from build123d import *

# Parameters (mm, degrees)
SKETCH1_W           = 10
SKETCH1_H           = 3
SKETCH1_W_2         = 3
SKETCH1_H_2         = 10
SKETCH1_R           = 3.25
BOSS_EXTRUDE1_DEPTH = 3


with BuildPart() as part:
    # Sketch1 → Boss-Extrude1 (new body)
    with BuildSketch(Plane.XY):
        Polygon((-112.631023813, -53.728350242), (-112.631023813, -63.840272517), (-112.631023813, -85.840272517), (119.257053912, -85.840272517), (137.368976187, -67.728350242), (187.368976187, -17.728350242), (137.368976187, 32.271649758), (137.368976187, 22.271649758), (134.368976187, 22.271649758), (134.368976187, 32.271649758), (60.378976187, 32.271649758), (60.378976187, 26.271649758), (57.378976187, 26.271649758), (57.378976187, 32.271649758), (42.378976187, 32.271649758), (27.378976187, 32.271649758), (27.378976187, 26.271649758), (24.378976187, 26.271649758), (24.378976187, 32.271649758), (-62.631023813, 32.271649758), (-109.631023813, 32.271649758), (-109.631023813, 22.271649758), (-112.631023813, 22.271649758), (-112.631023813, 12.271649758), (-109.631023813, 12.271649758), (-109.631023813, 2.271649758), (-112.631023813, 2.271649758), (-112.631023813, -7.728350242), (-109.631023813, -7.728350242), (-109.631023813, -17.728350242), (-112.631023813, -17.728350242), (-112.631023813, -27.728350242), (-109.631023813, -27.728350242), (-109.631023813, -50.728350242), (-102.631023813, -50.728350242), (-102.631023813, -53.728350242), align=None)
        with Locations((-87.631023813, -52.228350242)):
            Rectangle(SKETCH1_W, SKETCH1_H, mode=Mode.SUBTRACT)
        with Locations((-67.631023813, -52.228350242)):
            Rectangle(SKETCH1_W, SKETCH1_H, mode=Mode.SUBTRACT)
        with Locations((-47.631023813, -52.228350242)):
            Rectangle(SKETCH1_W, SKETCH1_H, mode=Mode.SUBTRACT)
        with Locations((-27.631023813, -52.228350242)):
            Rectangle(SKETCH1_W, SKETCH1_H, mode=Mode.SUBTRACT)
        with Locations((-7.631023813, -52.228350242)):
            Rectangle(SKETCH1_W, SKETCH1_H, mode=Mode.SUBTRACT)
        with Locations((12.368976187, -52.228350242)):
            Rectangle(SKETCH1_W, SKETCH1_H, mode=Mode.SUBTRACT)
        Polygon((27.368976187, -50.728350242), (37.371405326, -50.728350242), (37.368976187, -53.728350242), (27.368976187, -53.728350242), align=None, mode=Mode.SUBTRACT)
        Polygon((107.3787447, -50.728350242), (117.381121881, -50.728350242), (117.369073889, -53.728350242), (107.369073889, -53.728350242), align=None, mode=Mode.SUBTRACT)
        Polygon((127.381202522, -50.728350242), (137.381202522, -50.728350242), (137.36915453, -53.728350242), (127.36915453, -53.728350242), align=None, mode=Mode.SUBTRACT)
        with Locations((135.868976187, -32.728350242)):
            Rectangle(SKETCH1_W_2, SKETCH1_H_2, mode=Mode.SUBTRACT)
        with Locations((-57.669534365, 17.271649758)):
            Circle(SKETCH1_R, mode=Mode.SUBTRACT)
        with Locations((135.868976187, -12.728350242)):
            Rectangle(SKETCH1_W_2, SKETCH1_H_2, mode=Mode.SUBTRACT)
        with Locations((152.368976187, -17.728350242)):
            Rectangle(SKETCH1_W, SKETCH1_H, mode=Mode.SUBTRACT)
        with Locations((172.368976187, -17.728350242)):
            Rectangle(SKETCH1_W, SKETCH1_H, mode=Mode.SUBTRACT)
        with Locations((135.868976187, 7.271649758)):
            Rectangle(SKETCH1_W_2, SKETCH1_H_2, mode=Mode.SUBTRACT)
    extrude(amount=BOSS_EXTRUDE1_DEPTH)


solid = part.part
Build history of the part. All positions in model axes, mm. Round coordinates to 2 decimals unless told otherwise and drop trailing zeros. Loops run counter-clockwise (first coordinate to the right, second up) from the corner with the lowest first, then second, coordinate; pieces in that order, holes last. Notation, with made-up numbers: (29, 84.5) -> (84, 84.5) arc R5 ccw to (84, 90.5) -> close; hole circle Ø8 at (-8.5, -34). An arc over 180 degrees is marked (long way). One line per item, written item: value. Start each with the question number.
Q1. Drop flat-ended pins along their axis: pin 1 Ø1.5 at (x, z) = (130.5, 2) entering from -Y; pin 2 Ø0.9 at (x, z) = (172, 2) entering from +Y; pin 3 Ø1.5 at (y, z) = (-53, 1.5) entering from +X. Give the stop position or say it passes through.
Q2. Cut at C-C on z = 1. Count the separate pieces of the cut face and the enclosed holes in it, plus the area to 3 significant figures.
Q3. Probe line 1 along Y through (x, z) = (-9, 2.5); line 2 along X through (y, z) = (25, 1.5); line 3 along Y through (x, z) = (136, 2.7). List the from-to ranges inside material, lowest first.
Q4. Cut at D-D on y = -43. List the corners of the cut face in (x, z).
Q5. Cut at A-A on y = -31. List the corners of the cut face in (x, z), plus the area to 3 significant figures.
Q6. Two-plate mould, pull along Y, no slides. Class faces 1 (the face through (-60.249, 15.294, 1.479)), 2 (the face through (35, -26, 0)), 3 (the face through (162.72, 6.92, 1.48)), 4 (the face through (152.8, -52.3, 1.5)): released by +Y, released by -Y, zero draft, split by the parting line, or undercut.
Q7. Cut at B-B on y = 6. List the corners of the cut face in (x, z).
Computed:
1. pin 1: y = -75.35
1. pin 2: y = -1.91
1. pin 3: x = 152.85
2. separate pieces: 1
2. enclosed holes: 15
2. area: 31,200 mm²
3. line 1: -85.84 to -53.73, -50.73 to 32.27
3. line 2: -109.63 to 134.37, 137.37 to 144.64
3. line 3: -69.1 to -53.73, -50.73 to -37.73, -27.73 to -17.73, -7.73 to 2.27, 12.27 to 22.27
4. outline: (-109.63, 0) -> (162.1, 0) -> (162.1, 3) -> (-109.63, 3) -> close
5. outline: (-109.63, 0) -> (134.37, 0) -> (134.37, 3) -> (-109.63, 3) -> close; (137.37, 0) -> (174.1, 0) -> (174.1, 3) -> (137.37, 3) -> close
5. area: 842 mm²
6. face 1: undercut
6. face 2: zero draft
6. face 3: released by +Y
6. face 4: released by -Y
7. outline: (-109.63, 0) -> (134.37, 0) -> (134.37, 3) -> (-109.63, 3) -> close; (137.37, 0) -> (163.64, 0) -> (163.64, 3) -> (137.37, 3) -> close
